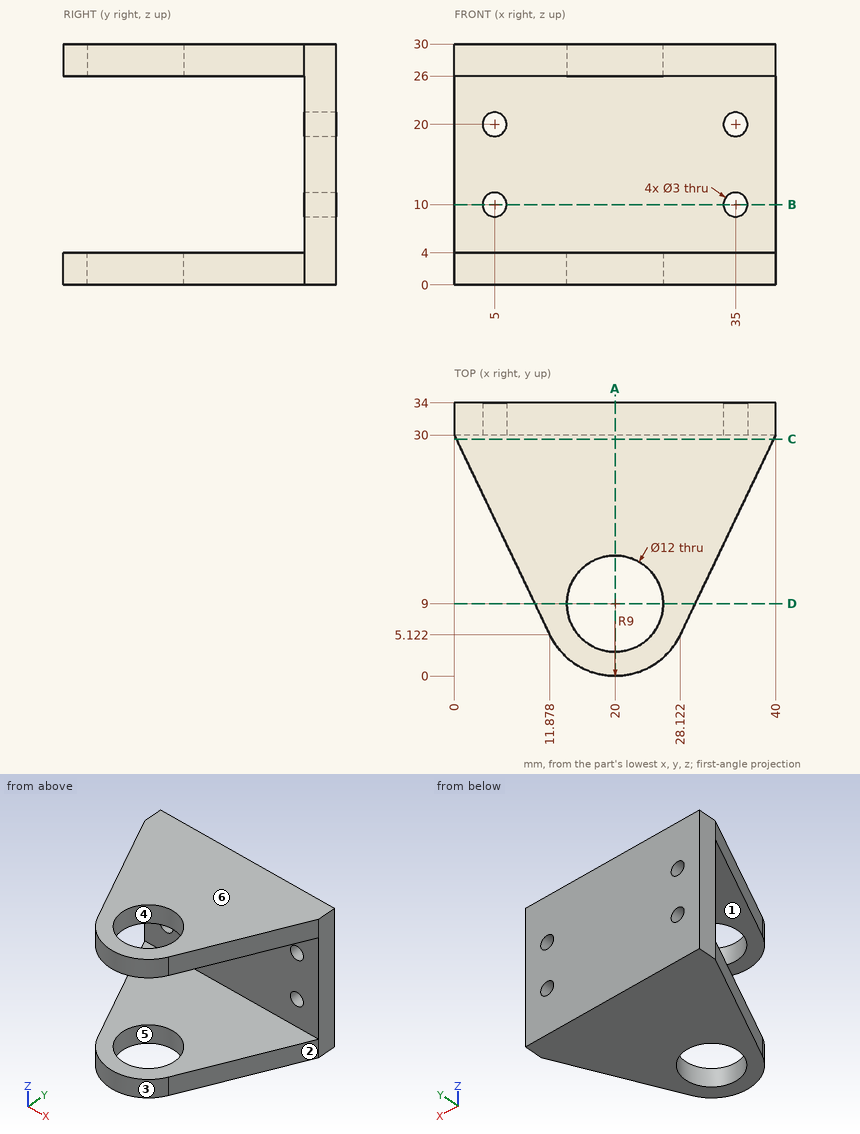
Input: dimensioned drawing with shaded views. Units: mm. Origin: part minimum x, y, z. A direction names the side the tool comes from. Coordinates: 2 decimals unless noted, no trailing zeros. Order: outer loops, then holes, each group sorted by start corner. A loop starts at its lowest first (then second) coordinate and runs counter-clockwise, first axis right, second up.
(1) Section query A-A (x = 20). Return the cut outline in (y, z).
(2) First-contact query: pin 1 (6 mm diameter, centred on x = 34, y = 17, fed in from +Z); pin 2 (5 mm diameter, centred on y = 6, z = 21.5, fed in from +X); pin 3 (10 mm diameter, centred on x = 35, z = 26, fed in from -Y) (1 decimal); pin 4 (3.5 mm diameter, centred on x = 35, z = 20, fed in from -Y). Flat tips, straight axial feed; report the tip coordinate or a pass-through.
(3) Access query for the marked faces 1 and 2. Directions: +Z, -Z, +X, -X, +Y, -Y. A direction counts if a zero-diameter tool reaches every point of the face in a straight line with its end or side. Return the directions, or none.
(4) Draft query along Y for the marked faces 3, 4, 5 and 6. Return one class per face: pulls with the +Y half, pulls with the -Y half, needs draft (parallel to the pull), parting line crosses it, or undercut.
(5) Section query D-D (y = 9). Return the cut outline in (x, z).
(6) Section query B-B (z = 10). Return the cut outline in (x, y).
(7) Section query C-C (y = 29.5). Return the cut outline in (x, z), plus the area to 3 significant figures.
(8) Material intervals for probe 1 along X at (y, z) = (32.5, 20); probe 2 along Z at (x, y) = (25.5, 4); probe 3 along X at (y, z) = (9, 28.8), sorted ascending.
Solution:
1. outline: (0, 0) - (3, 0) - (3, 4) - (0, 4) - close; (0, 26) - (3, 26) - (3, 30) - (0, 30) - close; (15, 0) - (34, 0) - (34, 30) - (15, 30) - (15, 26) - (30, 26) - (30, 4) - (15, 4) - close
2. pin 1: stops at z = 30
2. pin 2: passes through
2. pin 3: stops at y = 9.1
2. pin 4: stops at y = 30
3. face 1: +X, -X, -Y
3. face 2: +Z, -Z, +X, -Y
4. face 3: pulls with the -Y half
4. face 4: undercut
4. face 5: undercut
4. face 6: needs draft
5. outline: (10.03, 0) - (14, 0) - (14, 4) - (10.03, 4) - close; (10.03, 26) - (14, 26) - (14, 30) - (10.03, 30) - close; (26, 0) - (29.97, 0) - (29.97, 4) - (26, 4) - close; (26, 26) - (29.97, 26) - (29.97, 30) - (26, 30) - close
6. outline: (0, 30) - (3.5, 30) - (3.5, 34) - (0, 34) - close; (6.5, 30) - (33.5, 30) - (33.5, 34) - (6.5, 34) - close; (36.5, 30) - (40, 30) - (40, 34) - (36.5, 34) - close
7. outline: (0.24, 0) - (39.76, 0) - (39.76, 4) - (0.24, 4) - close; (0.24, 26) - (39.76, 26) - (39.76, 30) - (0.24, 30) - close
7. area: 316 mm2
8. probe 1: x = 0 to 3.5, 6.5 to 33.5, 36.5 to 40
8. probe 2: z = 0 to 4, 26 to 30
8. probe 3: x = 10.03 to 14, 26 to 29.97
